Can you work these out from the model? Positions are in its coordinate system, mm. Face numbers are marked on the shaded views. A direction names the side the tool comes from. Give positions to 0.01 mm unless a question says otherwise; leave off trailing zeros. Order: outer loops, then holes, each group sorted by start corner. A loop starts at its lowest first (then second) coordinate and runs counter-clockwise, first axis right, second up. Notation, with made-up numbers: M -11.75,-1 L 44.25,-1 A31 ccw 44.25,34 Z; hole C 89.25,59 d4. An arc over 180 degrees is marked long. Use one line per item in the form item = value. Start each with the question number.
1. I need wall thicknesses on L1, parallel to X at y = -6.5, z = 3.5; L2, parallel to Y at x = 8, z = -1; L3, parallel to Z at x = 17, y = 11.5. Which ranges of each line are inside material? Lowest first, please.
2. For the marked faces 4 and 5, which set-ups out of +Z, -Z, +X, -X, +Y, -Y let a thin tool reach every point of the face, with its end or its side?
3. I want a section at A-A, the plane x = 5.75. List the corners of the cut face in (y, z) for me, and give its area (3 significant figures).
4. I want a section at C-C, the plane z = 4.5. List the corners of the cut face in (x, y) for me.
5. Will these pins go through, and if not, where does the flat tip stop? P1, Ø4.5, axis at x = 11.5, y = 10.5, coming from the -Z side; P2, Ø8, axis at x = 2, y = 8, coming from the +Z side; P3, Ø0.8, axis at x = 10.5, z = 0.5, coming from the -Y side.
6. We'd pull the mould along X, two halves only. Please class the marked faces 1, 2 and 3: +X half, -X half, draft (parallel to the pull), parting line (faces both ways), or undercut.
7. I want a section at B-B, the plane y = -6. List the corners of the cut face in (x, z) for me, and give its area (3 significant figures).
8. I want a section at D-D, the plane x = 1.25. List the corners of the cut face in (y, z) for me.
```python
from build123d import *

# Parameters (mm, degrees)
SKIZZE1_W                       = 14.4
SKIZZE1_H                       = 16
AUFSATZ_LINEAR_AUSTRAGEN1_DEPTH = 1
AUFSATZ_LINEAR_AUSTRAGEN4_DEPTH = 15
SKIZZE9_W                       = 1.3
SKIZZE9_H                       = 13
AUFSATZ_LINEAR_AUSTRAGEN5_DEPTH = 2
SKIZZE10_W                      = 1
SKIZZE10_H                      = 16
AUFSATZ_LINEAR_AUSTRAGEN6_DEPTH = 5
SKIZZE13_W                      = 1
SKIZZE13_H                      = 16
SCHNITT_LINEAR_AUSTRAGEN4_DEPTH = 5


with BuildPart() as part:
    # Skizze1 → Aufsatz-Linear austragen1 (new body)
    with BuildSketch(Plane.XY):
        with Locations((7.2, 8)):
            Rectangle(SKIZZE1_W, SKIZZE1_H)
    extrude(amount=AUFSATZ_LINEAR_AUSTRAGEN1_DEPTH)

    # Skizze4 → Aufsatz-Linear austragen4 (add)
    with BuildSketch(Plane(origin=(14.4, 0, 0), x_dir=(0, 0, -1), z_dir=(1, 0, 0))):
        Polygon((0, 1.154700538), (0, 0), (1.5, -0.866025404), (-5, -12.124355653), (-4.133974596, -12.624355653), (2.866025404, -0.5), align=None)
    extrude(amount=-AUFSATZ_LINEAR_AUSTRAGEN4_DEPTH)

    # Skizze9 → Aufsatz-Linear austragen5 (add)
    with BuildSketch(Plane(origin=(0, -0.866025404, -1.5), x_dir=(1, 0, 0), z_dir=(0, 0.49999999999999484, 0.8660254037844418))):
        with Locations((13.75, -6.5)):
            Rectangle(SKIZZE9_W, SKIZZE9_H)
        with Locations((0.05, -6.5)):
            Rectangle(SKIZZE9_W, SKIZZE9_H)
    extrude(amount=AUFSATZ_LINEAR_AUSTRAGEN5_DEPTH)

    # Skizze10 → Aufsatz-Linear austragen6 (add)
    with BuildSketch(Plane(origin=(14.4, 0, 0), x_dir=(0, 0, -1), z_dir=(1, 0, 0))):
        with Locations((-0.5, 8)):
            Rectangle(SKIZZE10_W, SKIZZE10_H)
    extrude(amount=AUFSATZ_LINEAR_AUSTRAGEN6_DEPTH)

    # Skizze13 → Schnitt-Linear austragen4 (cut)
    with BuildSketch(Plane.ZY):
        with Locations((0.5, 8)):
            Rectangle(SKIZZE13_W, SKIZZE13_H)
    extrude(amount=-SCHNITT_LINEAR_AUSTRAGEN4_DEPTH, mode=Mode.SUBTRACT)


solid = part.part
```
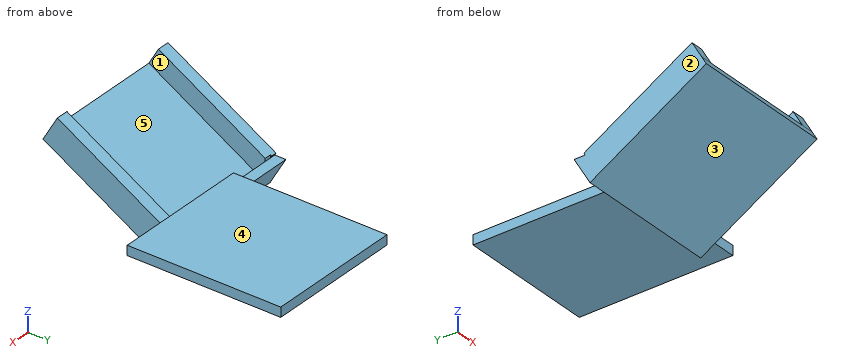
Check result:
q1.L1 = -0.6 to 0.7, 13.1 to 14.4
q1.L2 = -3.73 to -1.73, -0.58 to 0.58
q1.L3 = 0 to 1
q2.face_4 = +Z, +X, -X, +Y
q2.face_5 = +Z
q3.outline = M -12.62,4.13 L -0.5,-2.87 L 1.15,0 L 16,0 L 16,1 L 0,1 L 0,0 L -0.87,-1.5 L -12.12,5 Z
q3.area = 32.0 mm2
q4.outline = M -0.6,-12.41 L 14.4,-12.41 L 14.4,-7.26 L 13.1,-7.26 L 13.1,-11.26 L 0.7,-11.26 L 0.7,-7.26 L -0.6,-7.26 Z
q5.P1 = 0
q5.P2 = 1
q5.P3 = -7.02
q6.face_1 = undercut
q6.face_2 = -X half
q6.face_3 = draft
q7.outline = M -0.6,0.31 L 14.4,0.31 L 14.4,3.77 L 13.1,3.77 L 13.1,1.46 L 0.7,1.46 L 0.7,3.77 L -0.6,3.77 Z
q7.area = 23.3 mm2
q8.outline = M -12.62,4.13 L -0.5,-2.87 L 1.15,0 L 0,0 L -0.87,-1.5 L -12.12,5 Z
